Job drawing, mm, ordinate dimensions from the low corner. One solid piece. Round coordinates to 2 decimals unless told otherwise and drop trailing zeros. Write each loop counter-clockwise with the first axis right and the second up, starting at its lowest first coordinate (ties: lowest second). Pieces come first, ordered by that corner, then holes. Notation, with made-up numbers: M -5,3.5 L 37,3.5 A18 ccw 37,28.5 Z; hole C 18,20.5 d7. An arc over 180 degrees is marked long. Answer as a JSON object with one key per item and string values. Group by question number.
1. Drill centre lines: line 1 (X direction, y = 4.2, z = 15.25); line 2 (Z direction, x = 18, y = 3.1) (1 decimal); line 3 (Z direction, x = 21, y = 1.35) (1 decimal). Where is each one in solid material? Low to high. Write a range as from..to.
2. Two-plate mould, pull along X, no slides. Class the marked faces 1, 2 and 3: +X half, -X half, draft (parallel to the pull), parting line (faces both ways), or undercut.
3. Band-saw the part on A-A, the plane z = 17.75. Write the cut outline in (x, y) (1 decimal).
4. Band-saw the part on B-B, the plane x = 24.75. Write the cut outline in (y, z) (1 decimal).
5. Drop flat-ended pins along their axis: pin 1 (3 mm diameter, centred on y = 3, z = 17.5, fed in from -X); pin 2 (2.5 mm diameter, centred on x = 20.37, z = 23.67, fed in from -Y); pin 3 (4.5 mm diameter, centred on x = 19.82, z = 6.01, fed in from +Y); pin 4 (1.5 mm diameter, centred on x = 20, y = 2, fed in from -Z) (1 decimal). Give the stop position or say it passes through.
6. Band-saw the part on D-D, the plane x = 15. Write the cut outline in (y, z).
7. Band-saw the part on C-C, the plane y = 1.15. Count the separate pieces of the cut face and the enclosed holes in it, plus the area to 3 significant figures.
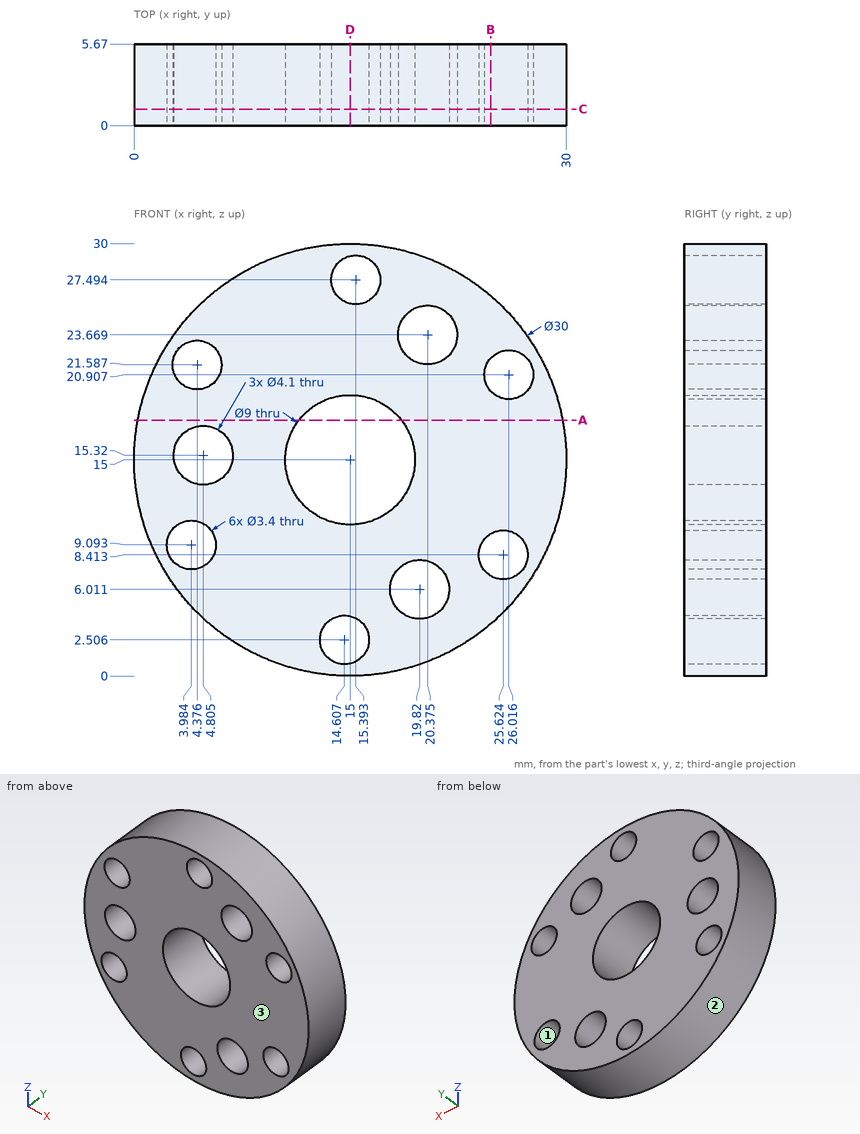
Worked answers:
{
 "1": {"line 1": "x = 0..2.76, 6.85..10.51, 19.49..30", "line 2": "z = 0.3..5.1, 7..11.6, 18.4..29.7", "line 3": "z = 1.3..4.3, 7.7..21.7, 25.6..28.7"},
 "2": {"face 1": "undercut", "face 2": "parting line", "face 3": "draft"},
 "3": {"outline": "M 0.3,0 L 11.4,0 L 11.4,5.7 L 0.3,5.7 Z; M 18.6,0 L 29.7,0 L 29.7,5.7 L 18.6,5.7 Z"},
 "4": {"outline": "M 0,3.6 L 5.7,3.6 L 5.7,7 L 0,7 Z; M 0,9.9 L 5.7,9.9 L 5.7,19.8 L 0,19.8 Z; M 0,22 L 5.7,22 L 5.7,26.4 L 0,26.4 Z"},
 "5": {"pin 1": "stops at x = 0.03", "pin 2": "passes through", "pin 3": "stops at y = 5.67", "pin 4": "stops at z = 0.6"},
 "6": {"outline": "M 0,0 L 5.67,0 L 5.67,0.85 L 0,0.85 Z; M 0,4.16 L 5.67,4.16 L 5.67,10.5 L 0,10.5 Z; M 0,19.5 L 5.67,19.5 L 5.67,25.84 L 0,25.84 Z; M 0,29.15 L 5.67,29.15 L 5.67,30 L 0,30 Z"},
 "7": {"separate pieces": "1", "enclosed holes": "10", "area": "549 mm^2"}
}
